```python
from build123d import *

# Parameters (mm, degrees)
EXTRUDE_1_DEPTH          = 3.5
SKETCH_2_R               = 19.5
EXTRUDE_2_DEPTH          = 7
PATTERN_CIRCULAR_1_COUNT = 22
SKETCH_3_R               = 16
CUT_EXTRUDE_1_DEPTH      = 2
SKETCH_4_R               = 16
EXTRUDE_3_DEPTH          = 3
SKETCH_5_R               = 6
EXTRUDE_4_DEPTH          = 2
SKETCH_6_R               = 2
EXTRUDE_5_DEPTH          = 3
SKETCH_7_R               = 5
EXTRUDE_6_DEPTH          = 2.5
EXTRUDE_7_DEPTH          = 10.5


with BuildPart() as part:
    # 草图1 → 凸台-拉伸1 (new, symmetric)
    with BuildSketch(Plane.XY):
        with BuildLine():
            ThreePointArc((1.077257951, 23.975811046), (-0.049799614, 21.8588225), (-0.453470023, 19.494726593))
            ThreePointArc((-0.453470023, 19.494726593), (1.390805461, 19.450338305), (3.222632926, 19.231865147))
            ThreePointArc((3.222632926, 19.231865147), (3.159441147, 21.629344251), (2.3450627, 23.885156079))
            ThreePointArc((2.3450627, 23.885156079), (1.711760568, 23.938877914), (1.077257951, 23.975811046))
        make_face()
    extrude_1 = extrude(amount=EXTRUDE_1_DEPTH, both=True)

    # 草图2 → 凸台-拉伸2 (add)
    with BuildSketch(Plane.XY.offset(3.5)):
        Circle(SKETCH_2_R)
    extrude(amount=-EXTRUDE_2_DEPTH)

    # 阵列(圆周)1: 凸台-拉伸1 ×22 about axis
    pattern_circular_1_axis = Axis((0, 0, 0), (0, 0, 1))
    for i in range(1, PATTERN_CIRCULAR_1_COUNT):
        add(extrude_1.rotate(pattern_circular_1_axis, i * 360 / PATTERN_CIRCULAR_1_COUNT))

    # 草图3 → 切除-拉伸1 (cut)
    with BuildSketch(Plane.XY.offset(3.5)):
        Circle(SKETCH_3_R)
    extrude(amount=-CUT_EXTRUDE_1_DEPTH, mode=Mode.SUBTRACT)

    # 草图4 → 凸台-拉伸3 (add)
    with BuildSketch(Plane(origin=(0, 0, -3.5), x_dir=(-1, 0, 0), z_dir=(0, 0, -1))):
        with Locations(Location((0, 0, 0), (0, 0, 180))):
            Circle(SKETCH_4_R)
    extrude(amount=EXTRUDE_3_DEPTH)

    # 草图5 → 凸台-拉伸4 (add)
    with BuildSketch(Plane(origin=(0, 0, -6.5), x_dir=(-1, 0, 0), z_dir=(0, 0, -1))):
        Circle(SKETCH_5_R)
    extrude(amount=EXTRUDE_4_DEPTH)

    # 草图6 → 凸台-拉伸5 (add)
    with BuildSketch(Plane(origin=(0, 0, -8.5), x_dir=(-1, 0, 0), z_dir=(0, 0, -1))):
        with BuildLine():
            Line((-3.730929356, 30.515982143), (-16.710418036, 11.268804464))
            ThreePointArc((-16.710418036, 11.268804464), (-20.155, 0), (-16.710418036, -11.268804464))
            Line((-16.710418036, -11.268804464), (-3.730929356, -30.515982143))
            ThreePointArc((-3.730929356, -30.515982143), (0, -32.5), (3.730929356, -30.515982143))
            Line((3.730929356, -30.515982143), (16.710418036, -11.268804464))
            ThreePointArc((16.710418036, -11.268804464), (20.155, 0), (16.710418036, 11.268804464))
            Line((16.710418036, 11.268804464), (3.730929356, 30.515982143))
            ThreePointArc((3.730929356, 30.515982143), (0, 32.5), (-3.730929356, 30.515982143))
        make_face()
        with Locations((0, 28)):
            Circle(SKETCH_6_R, mode=Mode.SUBTRACT)
        with Locations((0, -28)):
            Circle(SKETCH_6_R, mode=Mode.SUBTRACT)
    extrude(amount=EXTRUDE_5_DEPTH)

    # 草图7 → 凸台-拉伸6 (add)
    with BuildSketch(Plane(origin=(0, 0, -11.5), x_dir=(-1, 0, 0), z_dir=(0, 0, -1))):
        Circle(SKETCH_7_R)
    extrude(amount=EXTRUDE_6_DEPTH)

    # 草图8 → 凸台-拉伸7 (add)
    with BuildSketch(Plane.XY.offset(1.5)):
        Polygon((0, 7.505553499), (-6.5, 3.75277675), (-6.5, -3.75277675), (0, -7.505553499), (6.5, -3.75277675), (6.5, 3.75277675), align=None)
    extrude(amount=EXTRUDE_7_DEPTH)


solid = part.part
```
Work out the finished part from the listing and answer in its coordinate system (mm). A direction names the side the tool comes from. Coordinates: 2 decimals unless noted, no trailing zeros. Loops run counter-clockwise (first coordinate to the right, second up) from the corner with the lowest first, then second, coordinate; pieces in that order, holes last.
1) For faces 1 (the flat face through (10.31, -20.76, -9.98)), 2 (the cylindrical face through (-9.013, 19.879, 0.049)), 3 (the cylindrical face through (19.45, -1.4, 0.05)), determine the directions among +Z, -Z, +X, -X, +Y, -Y from which every point of the face is accessible in a straight line to the end or side of a thin tool.
Results:
face 1: -Z, +X, -Y
face 2: +Z, +Y
face 3: +Z, +X
2) Section B-B (z = 8.25) is taken. Give the vertices of the cut face in (x, y), plus the area to 3 significant figures.
Results:
outline: (-6.5, -3.75) - (0, -7.51) - (6.5, -3.75) - (6.5, 3.75) - (0, 7.51) - (-6.5, 3.75) - close
area: 146 mm2
3) Flat-ended cylindrical pins translate along their axes: pin 1 (1 mm diameter, centred on x = 4, y = -14, fed in from -Z); pin 2 (5 mm diameter, centred on y = 2.5, z = -3, fed in from -X); pin 3 (5 mm diameter, centred on y = 4.5, z = -4.5, fed in from +X). Find the tip coordinate at first contact, or state that the pin passes through.
Results:
pin 1: stops at z = -11.5
pin 2: stops at x = -23.58
pin 3: stops at x = 23.9
4) For a pull along X with two mould halves and no side action, classify faces 4 (the cylindrical face through (-6.13, -21.015, 0.049)), 5 (the cylindrical face through (-19.45, 1.4, 0.05)), 6 (the cylindrical face through (0.1, -32.5, -10)) as +X half, -X half, draft (parallel to the pull), parting line (faces both ways), or undercut.
Results:
face 4: undercut
face 5: -X half
face 6: parting line
5) Consider probe 1 along Z at (x, y) = (10, -2); probe 2 along Y at (x, z) = (14, 3.25); probe 3 along Z at (x, y) = (21, 3). Determine where each line is inside the solid, lowest interval first.
Results:
probe 1: z = -11.5 to -8.5, -6.5 to 1.5
probe 2: y = -16.38 to -7.75, 7.75 to 13.57, 15.74 to 19.49
probe 3: z = -3.5 to 3.5
6) Section A-A (y = 28) is taken. Give the vertices of the cut face in (x, z), plus the area to 3 significant figures.
Results:
outline: (-5.43, -11.5) - (-2, -11.5) - (-2, -8.5) - (-5.43, -8.5) - close; (2, -11.5) - (5.43, -11.5) - (5.43, -8.5) - (2, -8.5) - close
area: 20.6 mm2
